```python
from build123d import *

# Parameters (mm, degrees)
ESBO_O1_R                = 9.5
ESBO_O1_R_2              = 3
RESSALTO_EXTRUS_O1_DEPTH = 1.5
FILETE1_R                = 0.5
FILETE2_R                = 0.5
FILETE3_R                = 0.5


with BuildPart() as part:
    # Esboço1 → Ressalto-extrusão1 (new, symmetric)
    with BuildSketch(Plane.XY):
        Circle(ESBO_O1_R)
        Circle(ESBO_O1_R_2, mode=Mode.SUBTRACT)
    extrude(amount=RESSALTO_EXTRUS_O1_DEPTH, both=True)

    # Filete1
    filete1_edges = [part.edges().sort_by_distance(p)[0] for p in [
        (-9.5, 0, 1.5),
    ]]
    fillet(filete1_edges, radius=FILETE1_R)

    # Filete2
    filete2_edges = [part.edges().sort_by_distance(p)[0] for p in [
        (-9.5, 0, -1.5),
    ]]
    fillet(filete2_edges, radius=FILETE2_R)

    # Filete3
    filete3_edges = [part.edges().sort_by_distance(p)[0] for p in [
        (-3, 0, -1.5),
        (-3, 0, 1.5),
    ]]
    fillet(filete3_edges, radius=FILETE3_R)


solid = part.part
```
The listing builds one solid part. Answer for the finished solid, in the listing's coordinates (mm). Round coordinates to 2 decimals unless told otherwise and drop trailing zeros. Write each loop counter-clockwise with the first axis right and the second up, starting at its lowest first coordinate (ties: lowest second). Pieces come first, ordered by that corner, then holes. Notation, with made-up numbers: (77, 15) -> (110, 15) arc R21 ccw to (110, 25) -> close; hole circle Ø2 at (-1.75, 48.25). An arc over 180 degrees is marked (long way). Answer as a JSON object with one key per item and string values. Group by question number.
Q1. Section C-C (z = -0.6) is taken. Write down the section's boundary in (x, y), plus the area to 3 significant figures.
Q2. Section D-D (z = 1.25) is taken. Write down the section's boundary in (x, y).
Q3. This flat-tipped pin is pushed along its axis until it touches: pin 1 Ø1.5 at (y, z) = (-5.5, -0.5) entering from +X. Where does it stop, or does it pass through?
Q4. Straight lines are drawn through the part: line 1 along Y through (x, z) = (0, 0.4); line 2 along Y through (x, z) = (1, -0.95); line 3 along X through (y, z) = (1.5, -1.1). For each, find the intervals that lie inside material, in ascending order.
Q5. Section A-A (y = 0) is taken. Write down the section's boundary in (x, z), plus the area to 3 significant figures.
Q6. Determine the mould class of faces 1 (the face through (4.38, -8.43, 0.01)), 2 (the face through (-3, 0, 0)), 3 (the face through (0, -4, -1.5)) for opening direction X: pulls with the +X half, pulls with the -X half, needs draft (parallel to the pull), parting line crosses it, or undercut.
Check values:
{
 "1": {"outline": "circle Ø19 at (0, 0); hole circle Ø6 at (0, 0)", "area": "255 mm^2"},
 "2": {"outline": "circle Ø18.87 at (0, 0); hole circle Ø6.13 at (0, 0)"},
 "3": {"pin 1": "x = 8.23"},
 "4": {"line 1": "-9.5 to -3, 3 to 9.5", "line 2": "-9.45 to -2.83, 2.83 to 9.45", "line 3": "-9.37 to -2.61, 2.61 to 9.37"},
 "5": {"outline": "(-9.5, -1) arc R0.5 ccw to (-9, -1.5) -> (-3.5, -1.5) arc R0.5 ccw to (-3, -1) -> (-3, 1) arc R0.5 ccw to (-3.5, 1.5) -> (-9, 1.5) arc R0.5 ccw to (-9.5, 1) -> close; (3, -1) arc R0.5 ccw to (3.5, -1.5) -> (9, -1.5) arc R0.5 ccw to (9.5, -1) -> (9.5, 1) arc R0.5 ccw to (9, 1.5) -> (3.5, 1.5) arc R0.5 ccw to (3, 1) -> close", "area": "38.6 mm^2"},
 "6": {"face 1": "parting line crosses it", "face 2": "undercut", "face 3": "needs draft"}
}
